from build123d import *

# Parameters (mm, degrees)
BOSS_EXTRU_1_DEPTH = 5


with BuildPart() as part:
    # Esquisse2 → Boss.-Extru.1 (new body)
    with BuildSketch(Plane.XY):
        Polygon((-13.909341466, -8.713061229), (-12.409341466, -8.713061229), (-12.409341466, -18.713061229), (-8.409341466, -18.713061229), (-8.409341466, -8.713061229), (-4.409341466, -8.713061229), (-4.409341466, -18.713061229), (-0.409341466, -18.713061229), (-0.409341466, -8.713061229), (3.590658534, -8.713061229), (3.590658534, -18.713061229), (7.590658534, -18.713061229), (7.590658534, -8.713061229), (11.590658534, -8.713061229), (11.590658534, -18.713061229), (15.590658534, -18.713061229), (15.590658534, -6.213061229), (20.590658534, -6.213061229), (20.590658534, -1.213061229), (15.590658534, -1.213061229), (15.590658534, 3.786938771), (20.590658534, 3.786938771), (20.590658534, 8.786938771), (15.590658534, 8.786938771), (15.590658534, 18.786938771), (-13.909341466, 18.786938771), (-13.909341466, 8.786938771), (-18.909341466, 8.786938771), (-18.909341466, 3.786938771), (-13.909341466, 3.786938771), (-13.909341466, -1.213061229), (-18.909341466, -1.213061229), (-18.909341466, -6.213061229), (-13.909341466, -6.213061229), align=None)
    extrude(amount=BOSS_EXTRU_1_DEPTH)


solid = part.part
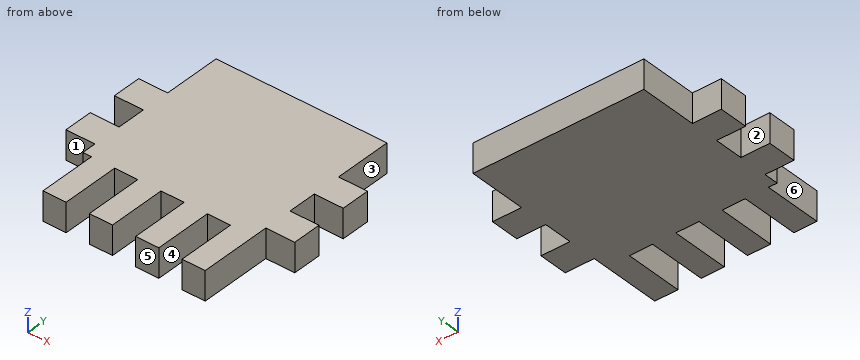
For this review, take the finished solid that the model builds, in its own axes (mm). Face numbers are marked on the shaded views. A direction names the side the tool comes from. Give positions to 0.01 mm unless a question says otherwise; leave off trailing zeros. Order: outer loops, then holes, each group sorted by start corner. A loop starts at its lowest first (then second) coordinate and runs counter-clockwise, first axis right, second up. Notation, with made-up numbers: M 7,27 L 55,27 A25 ccw 55,46 Z; hole C 61.5,55 d9. An arc over 180 degrees is marked long. Answer in a Markdown table with one row per item. Add a question column.
(1) For pin 1 (1.5 mm diameter, centred on y = -14.5, z = 2, fed in from +X); pin 2 (2 mm diameter, centred on x = 10, z = 3.5, fed in from -Y); pin 3 (1.5 mm diameter, centred on x = 17.5, z = 1.5, fed in from -Y), all flat-tipped, find the tip position at first contact; note any pin that passes through.
(2) For the marked faces 1, 2 and 3, list the 3-axis set-ups (+Z, -Z, +X, -X, +Y, -Y) from which the entire face can be reached by the end or side of a thin tool; tool diameter is ignored.
(3) Mouldability with a two-part tool opening along X and no side actions: class the marked faces 4, 5 and 6 as +X half, -X half, draft (parallel to the pull), parting line (faces both ways), or undercut.
(4) Consider section D-D on x = 9. State the section outline as (y, z) points, and give its area (4 significant figures).
(5) Wall thickness on probe 1 along X at (y, z) = (-14, 1.8); probe 2 along X at (y, z) = (-7.5, 0.65); probe 3 along Y at (x, z) = (-13, 4): over which ranges is each line inside the solid? List them lowest first. Write a range as [from, to].
(6) Consider section A-A on x = -14.5. State the section outline as (y, z) points, and give its area (3 significant figures).
(7) Consider section B-B on y = -13.5. State the section outline as (x, z) points, and give its area (3 significant figures).
Evaluation:
| question | item | result |
|---|---|---|
| 1 | pin 1 | stops at x = 15.59 |
| 1 | pin 2 | stops at y = -8.71 |
| 1 | pin 3 | stops at y = -6.21 |
| 2 | face 1 | +Z, -Z, -X, -Y |
| 2 | face 2 | +Z, -Z, -X |
| 2 | face 3 | +Z, -Z, +X, +Y |
| 3 | face 4 | undercut |
| 3 | face 5 | draft |
| 3 | face 6 | -X half |
| 4 | outline | M -8.71,0 L 18.79,0 L 18.79,5 L -8.71,5 Z |
| 4 | area | 137.5 mm^2 |
| 5 | probe 1 | x = [-12.41, -8.41], [-4.41, -0.41], [3.59, 7.59], [11.59, 15.59] |
| 5 | probe 2 | x = [-13.91, 15.59] |
| 5 | probe 3 | y = [-8.71, 18.79] |
| 6 | outline | M -6.21,0 L -1.21,0 L -1.21,5 L -6.21,5 Z; M 3.79,0 L 8.79,0 L 8.79,5 L 3.79,5 Z |
| 6 | area | 50.0 mm^2 |
| 7 | outline | M -12.41,0 L -8.41,0 L -8.41,5 L -12.41,5 Z; M -4.41,0 L -0.41,0 L -0.41,5 L -4.41,5 Z; M 3.59,0 L 7.59,0 L 7.59,5 L 3.59,5 Z; M 11.59,0 L 15.59,0 L 15.59,5 L 11.59,5 Z |
| 7 | area | 80.0 mm^2 |
